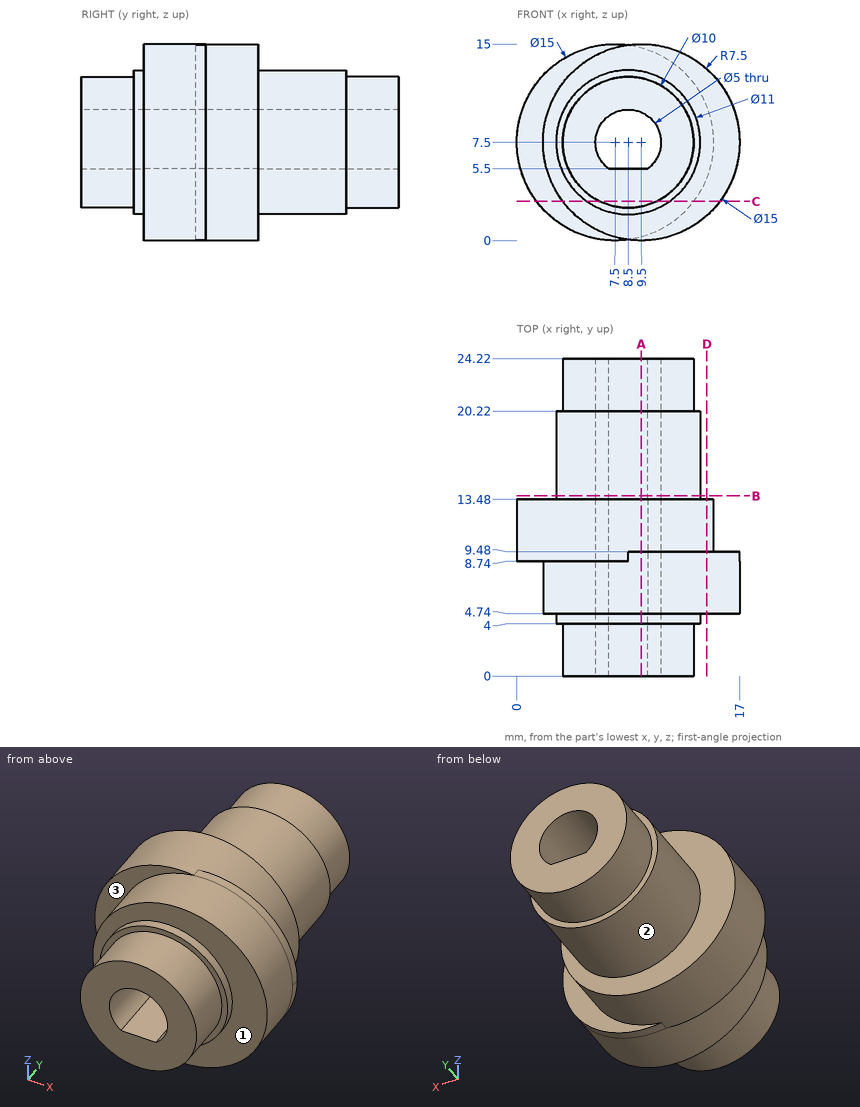
Design review of the part shown in the three views and the two pictorial views. Dimensions are in mm from the part's minimum x, y and z. A direction names the side the tool comes from. Round coordinates to 2 decimals unless told otherwise and drop trailing zeros. Write each loop counter-clockwise with the first axis right and the second up, starting at its lowest first coordinate (ties: lowest second). Pieces come first, ordered by that corner, then holes. Notation, with made-up numbers: (46.25, 66.5) -> (55.25, 66.5) arc R21 ccw to (55.25, 92.5) -> close; hole circle Ø7 at (0, 73.5). An arc over 180 degrees is marked (long way). Write item = value, one per line. Start each with the question number.
1) Take a section at D-D, the plane x = 14.5. State the section outline as (y, z) points, plus the area to 3 significant figures.
2) Take a section at A-A, the plane x = 9.5. State the section outline as (y, z) points, plus the area to 3 significant figures.
3) Tool access review of the marked faces 1, 2 and 3: name each direction out of +Z, -Z, +X, -X, +Y, -Y from which nothing blocks a thin tool from reaching the whole face with its end or side.
4) Clearance check with flat-ended pins moving along their axes: pin 1 (2 mm diameter, centred on y = 7.5, z = 7, fed in from -X); pin 2 (3 mm diameter, centred on x = 7.5, y = 20.5, fed in from +Z); pin 3 (1.5 mm diameter, centred on x = 8, y = 3, fed in from +Z); pin 4 (3 mm diameter, centred on x = 8.5, z = 7.5, fed in from +Y) (3 decimals). State where each tip first meets the part, or that it passes through.
5) Take a section at B-B, the plane y = 13.75. State the section outline as (x, z) points.
6) Wall thickness on probe 1 along X at (y, z) = (20.25, 7.5); probe 2 along Z at (x, y) = (8.5, 3); probe 3 along X at (y, z) = (19, 7.5): over which ranges is each line inside the solid? List them lowest first. Write a range as from..to.
7) Take a section at C-C, the plane z = 3. State the section outline as (x, y) points.
Results list:
q1.outline = (4.74, 1.91) -> (9.48, 1.91) -> (9.48, 4.81) -> (13.48, 4.81) -> (13.48, 10.19) -> (9.48, 10.19) -> (9.48, 13.09) -> (4.74, 13.09) -> close
q1.area = 74.5 mm²
q2.outline = (0, 2.6) -> (4, 2.6) -> (4, 2.09) -> (4.74, 2.09) -> (4.74, 0) -> (9.48, 0) -> (9.48, 0.27) -> (13.48, 0.27) -> (13.48, 2.09) -> (20.22, 2.09) -> (20.22, 2.6) -> (24.22, 2.6) -> (24.22, 5.5) -> (0, 5.5) -> close; (0, 9.79) -> (24.22, 9.79) -> (24.22, 12.4) -> (20.22, 12.4) -> (20.22, 12.91) -> (13.48, 12.91) -> (13.48, 14.73) -> (9.48, 14.73) -> (9.48, 15) -> (4.74, 15) -> (4.74, 12.91) -> (4, 12.91) -> (4, 12.4) -> (0, 12.4) -> close
q2.area = 184 mm²
q3.face_1 = -Y
q3.face_2 = +Y
q3.face_3 = -X, -Y
q4.pin_1 = 2
q4.pin_2 = 13
q4.pin_3 = 12.5
q4.pin_4 = through
q5.outline = circle Ø11 at (8.5, 7.5); hole (7, 5.5) -> (10, 5.5) arc R2.5 ccw (long way) to start
q6.probe_1 = 3.5..6, 11..13.5
q6.probe_2 = 2.5..5.5, 10..12.5
q6.probe_3 = 3..6, 11..14
q7.outline = (1.5, 8.74) -> (3.5, 8.74) -> (3.5, 4.74) -> (5.34, 4.74) -> (5.34, 4) -> (6.32, 4) -> (6.32, 0) -> (10.68, 0) -> (10.68, 4) -> (11.66, 4) -> (11.66, 4.74) -> (15.5, 4.74) -> (15.5, 9.48) -> (13.5, 9.48) -> (13.5, 13.48) -> (11.66, 13.48) -> (11.66, 20.22) -> (10.68, 20.22) -> (10.68, 24.22) -> (6.32, 24.22) -> (6.32, 20.22) -> (5.34, 20.22) -> (5.34, 13.48) -> (1.5, 13.48) -> close
